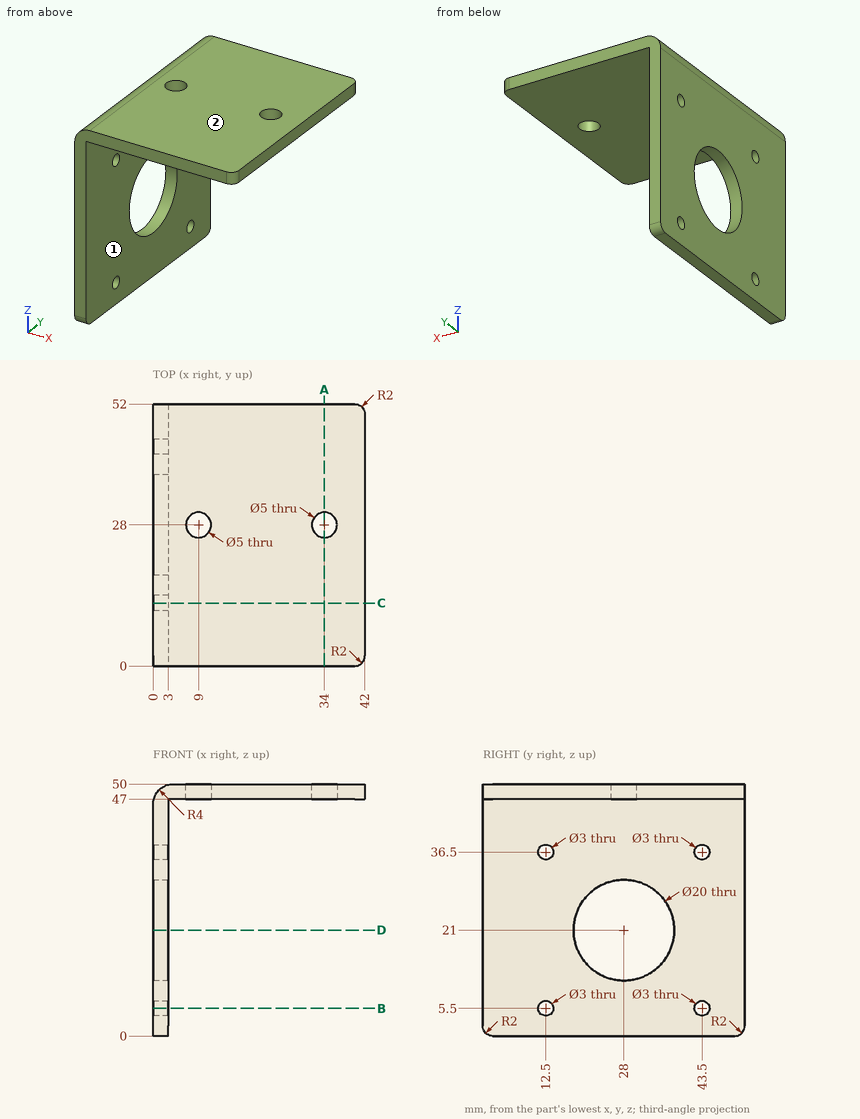
Geometry check sheet. Reference: drawing and pictorial views, mm from the part's lowest x, y, z. A direction names the side the tool comes from. Coordinates: 2 decimals unless noted, no trailing zeros. Order: outer loops, then holes, each group sorted by start corner. A loop starts at its lowest first (then second) coordinate and runs counter-clockwise, first axis right, second up. Notation, with made-up numbers: (84.25, -5.75) -> (127.25, -5.75) arc R19 ccw to (127.25, 31.25) -> close; hole circle Ø4 at (-19.75, 43.25). An arc over 180 degrees is marked (long way). Write item = value, one per line. Start each with the question number.
1) Cross-section at D-D (z = 21). Enter the section's corners in (x, y).
2) Access from +Z, -Z, +X, -X, +Y, -Y to the whole of each face (thin tool, end or side, straight path). Record for the marked faces 1 and 2.
3) Cross-section at B-B (z = 5.5). Enter the section's corners in (x, y), then the cut area to 3 significant figures.
4) Cross-section at A-A (x = 34). Enter the section's corners in (y, z).
5) Go/stop test with flat-tipped pins: P1, Ø5, axis at y = 12.5, z = 36.5, coming from the -X side; P2, Ø14, axis at y = 20, z = 31.5, coming from the +X side; P3, Ø10, axis at x = 27, y = 16.5, coming from the -Z side. Record where each tip stops, or that it passes through.
6) Material ranges on L1, parallel to Y at x = 0.9, z = 5.5; L2, parallel to Y at x = 9, z = 47.7; L3, parallel to Y at x = 1.2, z = 21, recorded low to high.
7) Cross-section at C-C (y = 12.5). Enter the section's corners in (x, z), then the cut area to 3 significant figures.
Ans:
q1.outline = (0, 0) -> (3, 0) -> (3, 18) -> (0, 18) -> close; (0, 38) -> (3, 38) -> (3, 52) -> (0, 52) -> close
q2.face_1 = -Z, +X, +Y, -Y
q2.face_2 = +Z, +X, -X, +Y, -Y
q3.outline = (0, 0) -> (3, 0) -> (3, 11) -> (0, 11) -> close; (0, 14) -> (3, 14) -> (3, 42) -> (0, 42) -> close; (0, 45) -> (3, 45) -> (3, 52) -> (0, 52) -> close
q3.area = 138 mm²
q4.outline = (0, 47) -> (25.5, 47) -> (25.5, 50) -> (0, 50) -> close; (30.5, 47) -> (52, 47) -> (52, 50) -> (30.5, 50) -> close
q5.P1 = 0
q5.P2 = 3
q5.P3 = 47
q6.L1 = 0 to 11, 14 to 42, 45 to 52
q6.L2 = 0 to 25.5, 30.5 to 52
q6.L3 = 0 to 18, 38 to 52
q7.outline = (0, 0) -> (3, 0) -> (3, 4) -> (0, 4) -> close; (0, 7) -> (3, 7) -> (3, 35) -> (0, 35) -> close; (0, 38) -> (3, 38) -> (3, 47) -> (42, 47) -> (42, 50) -> (4, 50) arc R4 ccw to (0, 46) -> close
q7.area = 246 mm²
